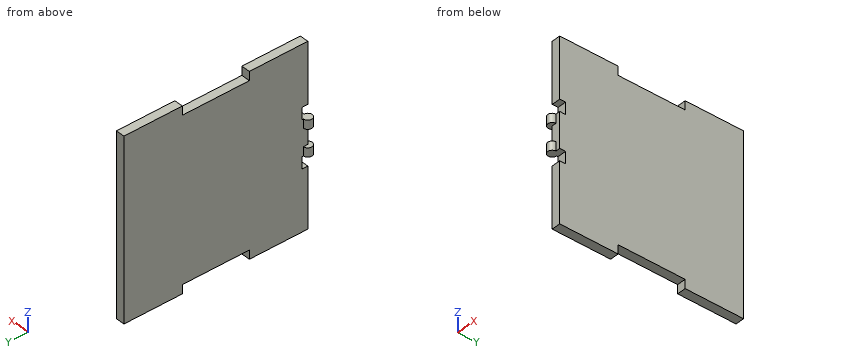
from build123d import *

# Parameters (mm, degrees)
BOSS_EXTRUDE1_DEPTH = 3
SKETCH4_R           = 1.5
BOSS_EXTRUDE2_DEPTH = 3
SKETCH5_W           = 4
SKETCH5_H           = 2
CUT_EXTRUDE1_DEPTH  = 10
LPATTERN1_COUNT     = 2
LPATTERN1_PITCH     = 9


with BuildPart() as part:
    # Sketch1 → Boss-Extrude1 (new body)
    with BuildSketch(Plane(origin=(0, 0, 0), x_dir=(0, 0, -1), z_dir=(1, 0, 0))):
        Polygon((-27.5, 0), (27.5, 0), (30.5, 0), (30.5, 20), (27.5, 20), (27.5, 42.94), (30.5, 42.94), (30.5, 62.94), (27.5, 62.94), (-27.5, 62.94), (-30.5, 62.94), (-30.5, 42.94), (-27.5, 42.94), (-27.5, 20), (-30.5, 20), (-30.5, 0), align=None)
    extrude(amount=BOSS_EXTRUDE1_DEPTH)

    # Sketch4 → Boss-Extrude2 (add)
    with BuildSketch(Plane.XY.offset(3)):
        Circle(SKETCH4_R)
    boss_extrude2 = extrude(amount=BOSS_EXTRUDE2_DEPTH)

    # Sketch5 → Cut-Extrude1 (cut)
    with BuildSketch(Plane.ZY):
        with Locations((-8, 1)):
            Rectangle(SKETCH5_W, SKETCH5_H)
        with Locations((8, 1)):
            Rectangle(SKETCH5_W, SKETCH5_H)
    extrude(amount=-CUT_EXTRUDE1_DEPTH, mode=Mode.SUBTRACT)

    # LPattern1: Boss-Extrude2 ×2
    with Locations(*[(0, 0, -i * LPATTERN1_PITCH) for i in range(1, LPATTERN1_COUNT)]):
        add(boss_extrude2)


solid = part.part
CAD build for the part. Positions are in the model's coordinates, mm. Give positions to 0.01 mm unless a question says otherwise; leave off trailing zeros. Loops run counter-clockwise (first coordinate to the right, second up) from the corner with the lowest first, then second, coordinate; pieces in that order, holes last. Notation, with made-up numbers: M 38,50 L 81,50 A23 cw 81,69 Z; hole C 53,13 d6. An arc over 180 degrees is marked long. Write each question's results on one line, items separated by ' | '.
Q1. Flat gauge pins, fed straight in: P1, Ø2, axis at x = 2, z = 17, coming from the -Y side; P2, Ø3, axis at y = 55.5, z = -11.5, coming from the -X side; P3, Ø0.9, axis at x = 1.5, z = -3, coming from the -Y side. Where does each tip first touch, or does it go through?
Geometry check:
P1: stops at y = 0 | P2: stops at x = 0 | P3: stops at y = -1.07
Q2. Band-saw the part on B-B on y = 35. Write the cut outline in (x, z), and give its area (3 significant figures).
Geometry check:
outline: M 0,-27.5 L 3,-27.5 L 3,27.5 L 0,27.5 Z | area: 165 mm²
Q3. Band-saw the part on A-A on y = 15. Write the cut outline in (x, z).
Geometry check:
outline: M 0,-30.5 L 3,-30.5 L 3,30.5 L 0,30.5 Z
Q4. Probe probe 1 along X at (y, z) = (17.5, -18); probe 2 along Y at (x, z) = (1.2, 19.5); probe 3 along Z at (x, y) = (1.65, 32). List the from-to ranges inside material, lowest first.
Geometry check:
probe 1: x = 0 to 3 | probe 2: y = 0 to 62.94 | probe 3: z = -27.5 to 27.5
